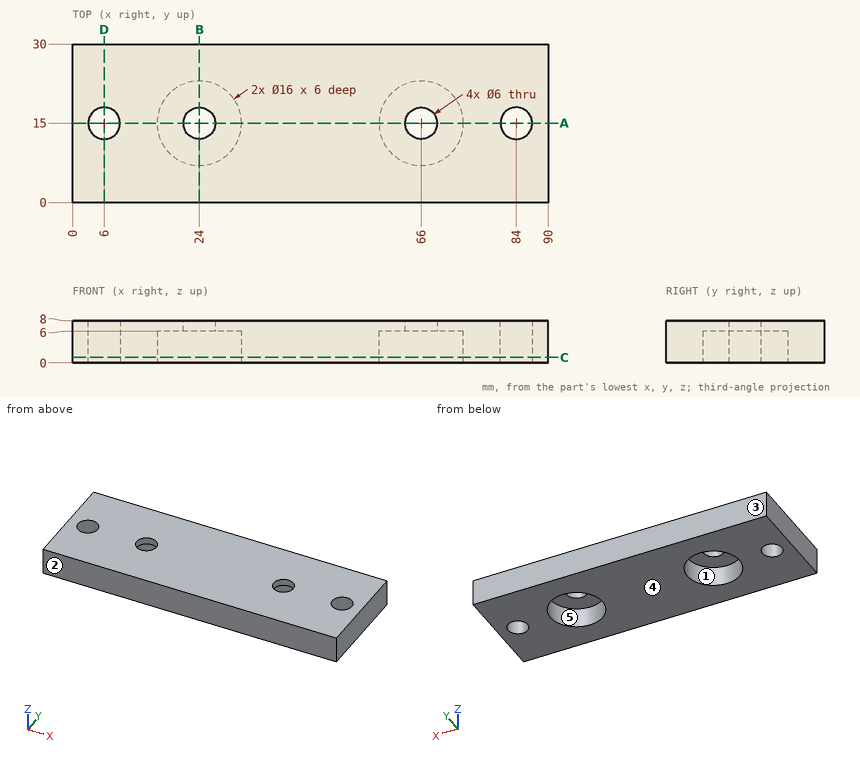
Could you check a few things on this drawing? It's one solid part, dimensions in mm from its lowest x, y, z. A direction names the side the tool comes from. Give positions to 0.01 mm unless a question says otherwise; leave off trailing zeros. Write each loop counter-clockwise with the first axis right and the second up, starting at its lowest first coordinate (ties: lowest second). Pieces come first, ordered by that corner, then holes.
(1) Imagine slicing it at C-C, the plane z = 1. Write out the boundary of the cut face in (x, y).
Output values:
outline: (0, 0) - (90, 0) - (90, 30) - (0, 30) - close; hole circle Ø6 at (6, 15); hole circle Ø16 at (24, 15); hole circle Ø16 at (66, 15); hole circle Ø6 at (84, 15)
(2) On a 3-axis mill with a long thin cutter (end or side, diameter ignored), from which of +Z, -Z, +X, -X, +Y, -Y can I reach the whole of each face in a straight line? I mean the marked faces 1 and 2. Say none if no direction works.
Output values:
face 1: -Z
face 2: +Z, -Z, +X, -X, -Y
(3) Will these pins go through, and if not, where does the flat tip stop? pin 1 (3.5 mm diameter, centred on x = 24, y = 15, fed in from +Z); pin 2 (8 mm diameter, centred on x = 66, y = 15, fed in from -Z).
Output values:
pin 1: passes through
pin 2: stops at z = 6
(4) Imagine slicing it at D-D, the plane x = 6. Write out the boundary of the cut face in (y, z).
Output values:
outline: (0, 0) - (12, 0) - (12, 8) - (0, 8) - close; (18, 0) - (30, 0) - (30, 8) - (18, 8) - close
(5) Thinking about a two-plate mould opening in Y: for the marked faces 3, 4 and 5, which applies, pulls with the +Y half, pulls with the -Y half, needs draft (parallel to the pull), parting line crosses it, or undercut?
Output values:
face 3: pulls with the +Y half
face 4: needs draft
face 5: undercut
(6) If I drill on L1, parallel to X at y = 15.25, z = 5.25; L2, parallel to X at y = 10.25, z = 3.25; L3, parallel to Y at x = 6, z = 4, over which ranges is the centre line in solid material (lowest first)?
Output values:
L1: x = 0 to 3.01, 8.99 to 16, 32 to 58, 74 to 81.01, 86.99 to 90
L2: x = 0 to 17.56, 30.44 to 59.56, 72.44 to 90
L3: y = 0 to 12, 18 to 30
(7) Imagine slicing it at A-A, the plane y = 15. Write out the boundary of the cut face in (x, z), and give its area (3 significant figures).
Output values:
outline: (0, 0) - (3, 0) - (3, 8) - (0, 8) - close; (9, 0) - (16, 0) - (16, 6) - (21, 6) - (21, 8) - (9, 8) - close; (27, 6) - (32, 6) - (32, 0) - (58, 0) - (58, 6) - (63, 6) - (63, 8) - (27, 8) - close; (69, 6) - (74, 6) - (74, 0) - (81, 0) - (81, 8) - (69, 8) - close; (87, 0) - (90, 0) - (90, 8) - (87, 8) - close
area: 408 mm2
(8) Imagine slicing it at B-B, the plane x = 24. Write out the boundary of the cut face in (y, z), and give its area (3 significant figures).
Output values:
outline: (0, 0) - (7, 0) - (7, 6) - (12, 6) - (12, 8) - (0, 8) - close; (18, 6) - (23, 6) - (23, 0) - (30, 0) - (30, 8) - (18, 8) - close
area: 132 mm2
